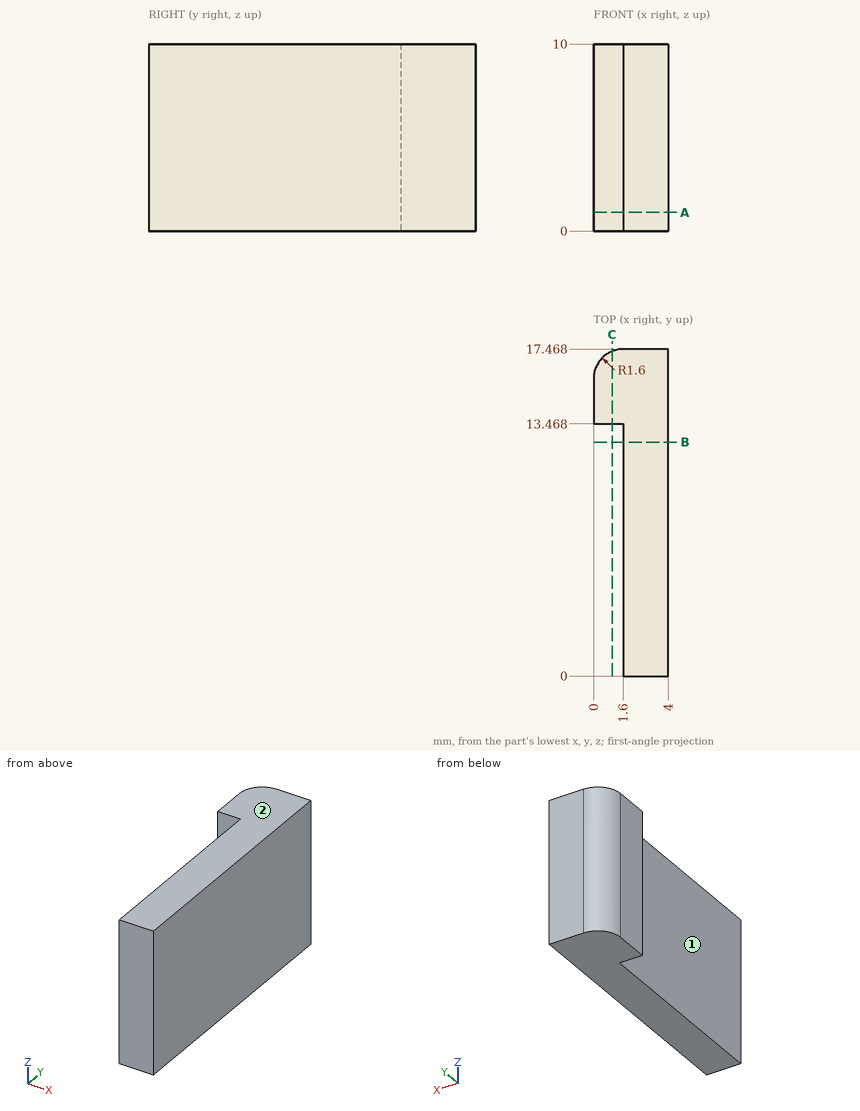
Input: dimensioned drawing with shaded views. Units: mm. Origin: part minimum x, y, z. A direction names the side the tool comes from. Give positions to 0.01 mm unless a question says otherwise; leave off trailing zeros. Write each loop counter-clockwise with the first axis right and the second up, starting at its lowest first coordinate (ties: lowest second). Pieces come first, ordered by that corner, then holes. Notation, with made-up numbers: M -1.75,2 L 14.25,2 A19 cw 14.25,21 Z; hole C 56,-11 d9. An arc over 180 degrees is marked long. Return JSON: item names as keys, results as strings. Group by question number.
1) Cut plane B-B, the plane y = 12.5. Output: boundary loops of the cut face in (x, z).
2) Material intervals for line 1 along X through (y, z) = (8, 8); line 2 along Y through (x, z) = (1.5, 5) (1 decimal); line 3 along Y through (x, z) = (1.35, 1.25), sorted ascending. Write a range as [from, to].
3) Cut plane A-A, the plane z = 1. Output: boundary loops of the cut face in (x, y), plus the area to 3 significant figures.
4) Cut plane C-C, the plane x = 1. Output: boundary loops of the cut face in (y, z), plus the area to 3 significant figures.
5) Set-up query: the marked faces 1 and 2. Return all of +Z, -Z, +X, -X, +Y, -Y with unobstructed straight access to the full face (end or side cutting, diameter ignored); none if empty.
6) Pin query (flat end, axial travel): P1, Ø2, axis at x = 0.5, y = 5.5, coming from the -Z side; P2, Ø5, axis at y = 3.5, z = 4, coming from the -X side; P3, Ø1.8, axis at x = 0.5, z = 5, coming from the -Y side. Return the tip coordinate at first contact, or that it passes through.
Recorded:
{
 "1": {"outline": "M 1.6,0 L 4,0 L 4,10 L 1.6,10 Z"},
 "2": {"line 1": "x = [1.6, 4]", "line 2": "y = [13.5, 17.5]", "line 3": "y = [13.47, 17.45]"},
 "3": {"outline": "M 0,13.47 L 1.6,13.47 L 1.6,0 L 4,0 L 4,17.47 L 1.6,17.47 A1.6 ccw 0,15.87 Z", "area": "47.8 mm²"},
 "4": {"outline": "M 13.47,0 L 17.35,0 L 17.35,10 L 13.47,10 Z", "area": "38.8 mm²"},
 "5": {"face 1": "+Z, -Z, -X, -Y", "face 2": "+Z, +X, -X, +Y, -Y"},
 "6": {"P1": "passes through", "P2": "stops at x = 1.6", "P3": "stops at y = 13.47"}
}
